```python
from build123d import *

# Parameters (mm, degrees)
F0_W     = 45.1445972584
F0_H     = 38.3139892519
F1_DEPTH = 2
F0_W_2   = 49.1445972584
F0_H_2   = 42.3139892519
F2_DEPTH = 25
F3_R     = 1.5
F4_DEPTH = 2


with BuildPart() as f1:
    # F0 (on Front) → F1 (new body)
    with BuildSketch(Plane.XZ):
        with Locations((0.661252765, 0)):
            Rectangle(F0_W, F0_H)
    extrude(amount=F1_DEPTH)

    # F0 (on Front) → F2 (join)
    with BuildSketch(Plane.XZ):
        with Locations((0.661252765, 0)):
            Rectangle(F0_W_2, F0_H_2)
        with Locations((0.661252765, 0)):
            Rectangle(F0_W, F0_H, mode=Mode.SUBTRACT)
    extrude(amount=F2_DEPTH)

    # F3 (on face) → F4 (cut, through all)
    with BuildSketch(Plane.YZ.offset(25.2335513942)):
        with Locations((-19.0394744277, -13.1474239752)):
            Circle(F3_R)
    extrude(amount=-F4_DEPTH, mode=Mode.SUBTRACT)


solid = f1.part
```
Model file for the job. Use its own axes, mm. A direction names the side the tool comes from. Give positions to 0.01 mm unless a question says otherwise; leave off trailing zeros. Order: outer loops, then holes, each group sorted by start corner. A loop starts at its lowest first (then second) coordinate and runs counter-clockwise, first axis right, second up.
1) Saw through at C-C, the plane x = 4.5. Write the cut outline in (y, z).
2) Saw through at D-D, the plane y = -18.25. Write the cut outline in (x, z).
3) 3-axis set-ups, long thin cutter, end or side, ignore diameter. For faces 5 (the flat face through (0, -13, 19.157)), 6 (the flat face through (0, 0, 0)): which of +Z, -Z, +X, -X, +Y, -Y reach the whole face in a straight line?
4) Mould opens along X. For faces 1 (the flat face through (25.234, -12, 0)), 2 (the flat face through (0, -13, -19.157)), 3 (the flat face through (-23.911, -12, 0)), 4 (the cylindrical face through (24.248, -17.609, -12.697)) say: +X half, -X half, draft (parallel to the pull), parting line (faces both ways), or undercut.
5) Saw through at A-A, the plane y = -7.75. Write the cut outline in (x, z), then the cut area to 3 significant figures.
6) Saw through at B-B, the plane z = -10.5. Write the cut outline in (x, y).
7) Wall check: probe 1 along X at (y, z) = (-8, -13); probe 2 along Z at (x, y) = (-13, -11); probe 3 along Y at (x, z) = (17.5, -18). Give the ranges that are in metal, low to high.
Computed:
1. outline: (-25, -21.16) - (0, -21.16) - (0, 21.16) - (-25, 21.16) - (-25, 19.16) - (-2, 19.16) - (-2, -19.16) - (-25, -19.16) - close
2. outline: (-23.91, -21.16) - (25.23, -21.16) - (25.23, -14.42) - (23.23, -14.42) - (23.23, -19.16) - (-21.91, -19.16) - (-21.91, 19.16) - (23.23, 19.16) - (23.23, -11.87) - (25.23, -11.87) - (25.23, 21.16) - (-23.91, 21.16) - close
3. face 5: -Y
3. face 6: +Z, -Z, +X, -X, +Y
4. face 1: +X half
4. face 2: undercut
4. face 3: -X half
4. face 4: draft
5. outline: (-23.91, -21.16) - (25.23, -21.16) - (25.23, 21.16) - (-23.91, 21.16) - close; hole (-21.91, -19.16) - (23.23, -19.16) - (23.23, 19.16) - (-21.91, 19.16) - close
5. area: 350 mm2
6. outline: (-23.91, -25) - (-21.91, -25) - (-21.91, -2) - (23.23, -2) - (23.23, -25) - (25.23, -25) - (25.23, 0) - (-23.91, 0) - close
7. probe 1: x = -23.91 to -21.91, 23.23 to 25.23
7. probe 2: z = -21.16 to -19.16, 19.16 to 21.16
7. probe 3: y = -2 to 0
